Input: part model. Units: mm. Frame: model coordinates. A direction names the side the tool comes from. Coordinates: 2 decimals unless noted, no trailing zeros. Order: outer loops, then holes, each group sorted by start corner. A loop starts at its lowest first (then second) coordinate and runs counter-clockwise, first axis right, second up. Notation, with made-up numbers: (20.5, -20.5) - (73.5, -20.5) arc R17 cw to (73.5, -8.5) - close; hole circle Ø9 at (41.25, 48.25). An arc over 180 degrees is marked (long way). Answer as CSV lines item,"result". Start each with the question number.
Item 1: First-contact query: pin 1 (5.5 mm diameter, centred on y = 5.5, z = -114.5, fed in from +X); pin 2 (7 mm diameter, centred on y = -4.5, z = -116, fed in from -X); pin 3 (0.7 mm diameter, centred on y = -8, z = -81, fed in from -X). Flat tips, straight axial feed; report the tip coordinate or a pass-through.
Item 2: Material intervals for line 1 along Y through (x, z) = (-1.5, -133) (3 decimals); line 2 along Y through (x, z) = (-5, -9); line 3 along X through (y, z) = (1.75, -19), sorted ascending.
Item 3: Access query for faces 1 (the flat face through (-1.016, -4, -110)), 2 (the flat face through (-5.334, 6, -110)), 3 (the flat face through (-4, 0, 0)). Directions: +Z, -Z, +X, -X, +Y, -Y. A direction counts if a zero-diameter tool reaches every point of the face in a straight line with its end or side. Return the directions, or none.
Item 4: Section B-B (y = 7.25). Output: boundary loops of the cut face in (x, z), and give its area (3 significant figures).
from build123d import *

# Parameters (mm, degrees)
EXTRUDE_THIN1_DEPTH = 222.25
FILLET1_R           = 1.016


with BuildPart() as part:
    # Sketch1 → Extrude-Thin1 (new body)
    with BuildSketch(Plane.XY):
        with BuildLine():
            Line((0, 0), (0, -9.525))
            Line((0, -9.525), (-3.175, -9.525))
            Line((-3.175, -9.525), (-3.175, -7.836680531))
            ThreePointArc((-3.175, -7.836680531), (-3.578277876, -4.661680531), (-4.7625, -1.688319469))
            Line((-4.7625, -1.688319469), (-4.7625, 0))
            Line((-4.7625, 0), (-6.35, 0))
            Line((-6.35, 0), (-6.35, 12.7))
            Line((-6.35, 12.7), (0, 12.7))
            Line((0, 12.7), (0, 11.684))
            Line((0, 11.684), (-5.334, 11.684))
            Line((-5.334, 11.684), (-5.334, 1.016))
            Line((-5.334, 1.016), (-3.7465, 1.016))
            Line((-3.7465, 1.016), (-3.7465, -1.431359013))
            ThreePointArc((-3.7465, -1.431359013), (-2.56178923, -4.537123743), (-2.159, -7.836680531))
            Line((-2.159, -7.836680531), (-2.159, -8.509))
            Line((-2.159, -8.509), (-1.016, -8.509))
            Line((-1.016, -8.509), (-1.016, 0))
            Line((-1.016, 0), (0, 0))
        make_face()
    extrude(amount=-EXTRUDE_THIN1_DEPTH)

    # Fillet1
    fillet1_edges = [part.edges().sort_by_distance(p)[0] for p in [
        (-3.7465, 1.016, -111.125),
        (0, -9.525, -111.125),
        (-3.175, -9.525, -111.125),
        (-4.7625, -1.688319469, -111.125),
        (-6.35, 0, -111.125),
        (-6.35, 12.7, -111.125),
    ]]
    fillet(fillet1_edges, radius=FILLET1_R)


solid = part.part
Determined:
1,pin 1,"stops at x = -5.33"
1,pin 2,"stops at x = -4.76"
1,pin 3,"stops at x = -3.18"
2,line 1,"y = -9.525 to -8.509, 11.684 to 12.7"
2,line 2,"y = 0 to 1.02, 11.68 to 12.7"
2,line 3,"x = -6.35 to -5.33"
3,face 1,"+Z, -Z"
3,face 2,"+Z, -Z, +X"
3,face 3,"+Z, +X, -X, +Y, -Y"
4,outline,"(-6.35, -222.25) - (-5.33, -222.25) - (-5.33, 0) - (-6.35, 0) - close"
4,area,"226 mm^2"
